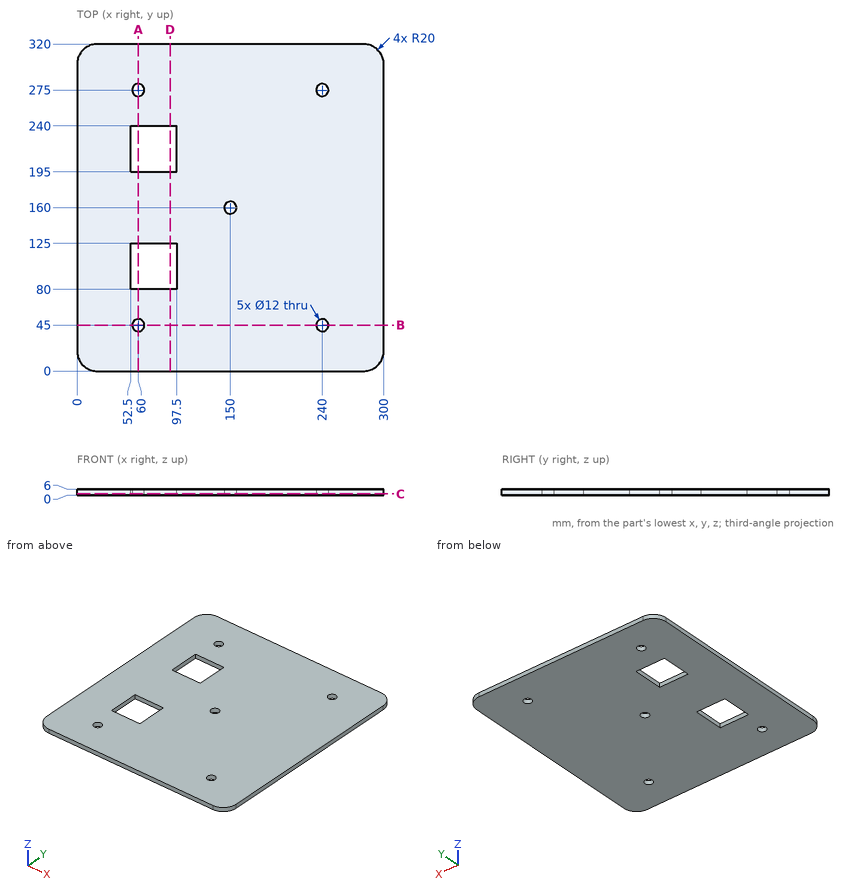
Study the drawing (mm; zero at the part's minimum x, y, z) and answer. Coordinates: 2 decimals unless noted, no trailing zeros. Loops run counter-clockwise (first coordinate to the right, second up) from the corner with the lowest first, then second, coordinate; pieces in that order, holes last. Notation, with made-up numbers: M 22,-6.75 L 81,-6.75 A27 ccw 81,25.25 Z; hole C -22,54.5 d11. An arc over 180 degrees is marked long. Answer in a Markdown table with one row per item. Add a question column.
1. Find section A-A, the plane x = 60. Write down the section's boundary in (y, z).
2. Find section C-C, the plane z = 1.5. Write down the section's boundary in (x, y), then the cut area to 3 significant figures.
3. Consider L1, parallel to Y at x = 60, z = 1.8; L2, parallel to Y at x = 240, z = 1.55; L3, parallel to Y at x = 78.5, z = 3.8. Determine where each line is inside the solid, lowest interval first.
4. Find section B-B, the plane y = 45. Write down the section's boundary in (x, z), then the cut area to 3 significant figures.
5. Find section D-D, the plane x = 91. Write down the section's boundary in (y, z).
Reported:
| question | item | result |
|---|---|---|
| 1 | outline | M 0,0 L 39,0 L 39,6 L 0,6 Z; M 51,0 L 80,0 L 80,6 L 51,6 Z; M 125,0 L 195,0 L 195,6 L 125,6 Z; M 240,0 L 269,0 L 269,6 L 240,6 Z; M 281,0 L 320,0 L 320,6 L 281,6 Z |
| 2 | outline | M 0,20 A20 ccw 20,0 L 280,0 A20 ccw 300,20 L 300,300 A20 ccw 280,320 L 20,320 A20 ccw 0,300 Z; hole M 52.5,80 L 97.5,80 L 97.5,125 L 52.5,125 Z; hole M 52.5,195 L 97.5,195 L 97.5,240 L 52.5,240 Z; hole C 60,45 d12; hole C 60,275 d12; hole C 150,160 d12; hole C 240,45 d12; hole C 240,275 d12 |
| 2 | area | 91,000 mm^2 |
| 3 | L1 | y = 0 to 39, 51 to 80, 125 to 195, 240 to 269, 281 to 320 |
| 3 | L2 | y = 0 to 39, 51 to 269, 281 to 320 |
| 3 | L3 | y = 0 to 80, 125 to 195, 240 to 320 |
| 4 | outline | M 0,0 L 54,0 L 54,6 L 0,6 Z; M 66,0 L 234,0 L 234,6 L 66,6 Z; M 246,0 L 300,0 L 300,6 L 246,6 Z |
| 4 | area | 1,660 mm^2 |
| 5 | outline | M 0,0 L 80,0 L 80,6 L 0,6 Z; M 125,0 L 195,0 L 195,6 L 125,6 Z; M 240,0 L 320,0 L 320,6 L 240,6 Z |
